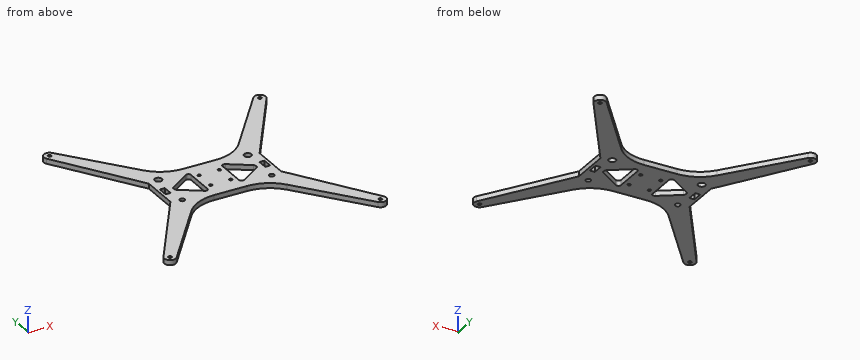
from build123d import *

# Parameters (mm, degrees)
F0_R     = 1.65
F0_R_2   = 2.55
F0_W     = 5
F0_H     = 10
F0_R_3   = 1.5
F0_R_4   = 3.555
F1_DEPTH = 5


# Not quite as in the source:
# - ends of sketch curves that miss each other by under 0.0002 mm in the source are joined


with BuildPart() as f1:
    # F0 (on Top) → F1 (new body)
    with BuildSketch(Plane.XY):
        with BuildLine():
            Line((-47.640397, 42.115595), (-100.031737, 108.050449))
            ThreePointArc((-100.031737, 108.050449), (-107.8442155419, 109.1246397394), (-109.2715048598, 101.368896092))
            Line((-109.2715048598, 101.368896092), (-54.999977, 18.664241))
            Line((-54.999977, 18.664241), (-54.999977, -18.664242))
            Line((-54.999977, -18.664242), (-109.271505, -101.368897))
            ThreePointArc((-109.271505, -101.368897), (-107.8441644553, -109.1246766812), (-100.031658534, -108.0503513703))
            Line((-100.031658534, -108.0503513703), (-47.643302, -42.116283))
            ThreePointArc((-47.643302, -42.116283), (-33.7130803066, -30.9767526972), (-16.325566, -27))
            Line((-16.325566, -27), (16.325565, -27))
            ThreePointArc((16.325565, -27), (33.7130793066, -30.9767526972), (47.6433013924, -42.1162826882))
            Line((47.6433013924, -42.1162826882), (100.031658, -108.050351))
            ThreePointArc((100.031658, -108.050351), (107.8441644255, -109.1246767027), (109.2715050175, -101.3688963323))
            Line((109.2715050175, -101.3688963323), (54.999976, -18.664242))
            Line((54.999976, -18.664242), (54.999976, 18.664241))
            Line((54.999976, 18.664241), (109.271504, 101.368896))
            ThreePointArc((109.271504, 101.368896), (107.8442155121, 109.1246397609), (100.0317360662, 108.0504489474))
            Line((100.0317360662, 108.0504489474), (47.640396, 42.115595))
            ThreePointArc((47.640396, 42.115595), (33.7103248028, 30.9765618002), (16.323206, 27))
            Line((16.323206, 27), (-16.323206, 27))
            ThreePointArc((-16.323206, 27), (-33.710325083, 30.9765619354), (-47.640397, 42.115595))
        make_face()
        with Locations((-104.5, -104.5)):
            Circle(F0_R, mode=Mode.SUBTRACT)
        with Locations((-44.444977, -20.807752)):
            Circle(F0_R_2, mode=Mode.SUBTRACT)
        with Locations((-49.499977, 0)):
            Rectangle(F0_W, F0_H, mode=Mode.SUBTRACT)
        with BuildLine():
            Line((-19.581953, -16.373154), (-39.803759, -2.743263))
            ThreePointArc((-39.803759, -2.743263), (-40.6136447533, -1.8442487652), (-40.906473, -0.670199))
            Line((-40.906473, -0.670199), (-40.906473, 0.670176))
            ThreePointArc((-40.906473, 0.670176), (-40.6136450793, 1.8442251525), (-39.8037598701, 2.7432388072))
            Line((-39.8037598701, 2.7432388072), (-19.581955, 16.373149))
            ThreePointArc((-19.581955, 16.373149), (-17.0106188475, 16.5072580793), (-15.684668, 14.300086))
            Line((-15.684668, 14.300086), (-15.684668, -14.30009))
            ThreePointArc((-15.684668, -14.30009), (-17.0106178687, -16.5072615586), (-19.581953, -16.373154))
        make_face(mode=Mode.SUBTRACT)
        with Locations((-10, -10)):
            Circle(F0_R_3, mode=Mode.SUBTRACT)
        with Locations((104.5, -104.5)):
            Circle(F0_R, mode=Mode.SUBTRACT)
        with Locations((10, -10)):
            Circle(F0_R_3, mode=Mode.SUBTRACT)
        with Locations((44.444976, -20.807752)):
            Circle(F0_R_2, mode=Mode.SUBTRACT)
        with BuildLine():
            Line((19.581954, 16.373149), (39.803759, 2.743239))
            ThreePointArc((39.803759, 2.743239), (40.6136440793, 1.8442251525), (40.906472, 0.670176))
            Line((40.906472, 0.670176), (40.906472, -0.670199))
            ThreePointArc((40.906472, -0.670199), (40.6136437533, -1.8442487652), (39.803757719, -2.7432625831))
            Line((39.803757719, -2.7432625831), (19.581952, -16.373154))
            ThreePointArc((19.581952, -16.373154), (17.0106168687, -16.5072615586), (15.684667, -14.30009))
            Line((15.684667, -14.30009), (15.684667, 14.300086))
            ThreePointArc((15.684667, 14.300086), (17.0106178475, 16.5072580793), (19.581954, 16.373149))
        make_face(mode=Mode.SUBTRACT)
        with Locations((49.499976, 0)):
            Rectangle(F0_W, F0_H, mode=Mode.SUBTRACT)
        with Locations((-44.444977, 20.810818)):
            Circle(F0_R_4, mode=Mode.SUBTRACT)
        with Locations((-10, 10)):
            Circle(F0_R_3, mode=Mode.SUBTRACT)
        with Locations((-104.5, 104.5)):
            Circle(F0_R, mode=Mode.SUBTRACT)
        with Locations((10, 10)):
            Circle(F0_R_3, mode=Mode.SUBTRACT)
        with Locations((44.444976, 20.810818)):
            Circle(F0_R_4, mode=Mode.SUBTRACT)
        with Locations((104.5, 104.5)):
            Circle(F0_R, mode=Mode.SUBTRACT)
    extrude(amount=F1_DEPTH)


solid = f1.part
Input: part model. Units: mm. Frame: model coordinates. Give positions to 0.01 mm unless a question says otherwise; leave off trailing zeros. Write each loop counter-clockwise with the first axis right and the second up, starting at its lowest first coordinate (ties: lowest second). Pieces come first, ordered by that corner, then holes. Notation, with made-up numbers: M 70,-33.75 L 77,-33.75 A9 cw 77,-25.75 Z; hole C 49.5,74.25 d3. An arc over 180 degrees is marked long. Write item = value, one per line. Start each with the question number.
1) Cut plane B-B on x = -93. Return the cut outline in (y, z).
2) First-contact query: pin 1 Ø1.5 at (x, z) = (62.5, 1.5) entering from -Y; pin 2 Ø1.5 at (x, z) = (75, 2) entering from +Y; pin 3 Ø2 at (y, z) = (-43.5, 2.5) entering from +X. Flat tips, straight axial feed; report the tip coordinate or a pass-through.
3) Cut plane C-C on z = 3.9. Count the separate pieces of the cut face and the enclosed holes in it, then the cut area to 3 significant figures.
4) Material intervals for line 1 along Y through (x, z) = (-10, 3.55); line 2 along X through (y, z) = (104.5, 3.2); line 3 along Y through (x, z) = (-104.5, 1.2), sorted ascending. Write a range as [from, to].
5) Cut plane A-A on y = 77.5. Return the cut outline in (x, z).
Solved:
q1.outline = M -99.2,0 L -76.57,0 L -76.57,5 L -99.2,5 Z; M 76.57,0 L 99.2,0 L 99.2,5 L 76.57,5 Z
q2.pin_1 = -61.76
q2.pin_2 = 77.49
q2.pin_3 = 71.95
q3.separate_pieces = 1
q3.enclosed_holes = 16
q3.area = 11,200 mm2
q4.line_1 = [-27, -11.5], [-8.5, 8.5], [11.5, 27]
q4.line_2 = [-110.21, -106.15], [-102.85, -97.21], [97.21, 102.85], [106.15, 110.21]
q4.line_3 = [-110.21, -106.15], [-102.85, -94.1], [94.1, 102.85], [106.15, 110.21]
q5.outline = M -93.61,0 L -75.76,0 L -75.76,5 L -93.61,5 Z; M 75.76,0 L 93.61,0 L 93.61,5 L 75.76,5 Z
